Build history of the part. All positions in model axes, mm. A direction names the side the tool comes from. Give positions to 0.01 mm unless a question says otherwise; leave off trailing zeros. Order: outer loops, then holes, each group sorted by start corner. A loop starts at its lowest first (then second) coordinate and runs counter-clockwise, first axis right, second up. Notation, with made-up numbers: (-25.75, 23) -> (-10.75, 23) arc R22 ccw to (-10.75, 43) -> close; hole circle Ø9 at (28, -8). An arc over 180 degrees is marked (long way). One line per item, written item: value. Start each with the question number.
(1) Saw through at C-C on x = -5. Give the cut face in (y, z).
(2) Saw through at B-B on x = 5.5. Give the cut face in (y, z).
(3) Pin check, flat tips, straight feed: pin 1 (1.8 mm diameter, centred on x = 15.5, y = -1, fed in from +Z); pin 2 (10 mm diameter, centred on y = -3, z = 33, fed in from +X); pin 3 (3 mm diameter, centred on y = 1.5, z = 20.5, fed in from +X). Stop position of each tip, or through.
(4) Two-plate mould, pull along Y, no slides. Class faces 6 (the flat face through (6, 0, 19.55)), 7 (the flat face through (5, 0, 23)), 8 (the flat face through (0, 10, 6)): +Y half, -Y half, draft (parallel to the pull), parting line (faces both ways), or undercut.
(5) Saw through at D-D on z = 23.5. Give the cut face in (x, y), plus the area to 3 significant figures.
(6) Probe line 1 (X direction, y = 0, z = 1.7); line 2 (Y direction, x = -5, z = 3); line 3 (X direction, y = 4.5, z = 32). List the from-to ranges inside material, lowest first.
(7) Which spindle directions (+Z, -Z, +X, -X, +Y, -Y) get a long thin tool onto all of the face, cutting with end or side? Do faces 1 (the cylindrical face through (12.789, 1.933, 6.521)), 2 (the flat face through (-10, 0, 23)), 3 (the flat face through (15.437, 7.535, 23.21)), 4 (the flat face through (6, 0, 12.45)), 5 (the flat face through (18.4, 0.1, 8)). Say none if no direction does.
(8) Saw through at A-A on z = 30.5. Give the cut face in (x, y).
```python
from build123d import *

# Parameters (mm, degrees)
SKETCH1_W           = 40
SKETCH1_H           = 20
SKETCH1_R           = 1.65
BOSS_EXTRUDE1_DEPTH = 8
SKETCH3_W           = 3
SKETCH3_H           = 20
SKETCH3_W_2         = 6
BOSS_EXTRUDE2_DEPTH = 30
BOSS_EXTRUDE3_DEPTH = 20
SKETCH6_W           = 7
SKETCH6_H           = 10
SKETCH6_W_2         = 9
CUT_EXTRUDE2_DEPTH  = 30
SKETCH7_R           = 2.15
CUT_EXTRUDE3_DEPTH  = 6
CUT_EXTRUDE4_DEPTH  = 2.5
SKETCH10_R          = 3
CUT_EXTRUDE5_DEPTH  = 3


with BuildPart() as part:
    # Sketch1 → Boss-Extrude1 (new body)
    with BuildSketch(Plane.XY):
        Rectangle(SKETCH1_W, SKETCH1_H)
        with Locations((-5, 0)):
            Circle(SKETCH1_R, mode=Mode.SUBTRACT)
        with Locations((14.999778189, -0.094193404)):
            Circle(SKETCH1_R, mode=Mode.SUBTRACT)
    extrude(amount=BOSS_EXTRUDE1_DEPTH)

    # Sketch3 → Boss-Extrude2 (add)
    with BuildSketch(Plane.XY.offset(8)):
        with Locations((-11.5, 0)):
            Rectangle(SKETCH3_W, SKETCH3_H)
        with Locations((8, 0)):
            Rectangle(SKETCH3_W_2, SKETCH3_H)
    extrude(amount=BOSS_EXTRUDE2_DEPTH)

    # Sketch5 → Boss-Extrude3 (add)
    with BuildSketch(Plane(origin=(0, 10, 0), x_dir=(1, 0, 0), z_dir=(0, 1, 0))):
        Polygon((-20, -8), (-13, -38), (-13, -8), align=None)
        Polygon((20, -8), (11, -8), (11, -38), align=None)
    extrude(amount=-BOSS_EXTRUDE3_DEPTH)

    # Sketch6 → Cut-Extrude2 (cut)
    with BuildSketch(Plane.XY.offset(38)):
        with Locations((-16.5, 0)):
            Rectangle(SKETCH6_W, SKETCH6_H)
        with Locations((15.5, 0)):
            Rectangle(SKETCH6_W_2, SKETCH6_H)
    extrude(amount=-CUT_EXTRUDE2_DEPTH, mode=Mode.SUBTRACT)

    # Sketch7 → Cut-Extrude3 (cut)
    with BuildSketch(Plane(origin=(11, 0, 0), x_dir=(0, 0, -1), z_dir=(1, 0, 0))):
        with Locations(Location((-16, 0, 0), (0, 0, 90))):
            Circle(SKETCH7_R)
    extrude(amount=-CUT_EXTRUDE3_DEPTH, mode=Mode.SUBTRACT)

    # Sketch8 → Cut-Extrude4 (cut)
    with BuildSketch(Plane.ZY.offset(-5)):
        Polygon((19.55, 2.049593456), (16, 4.099186911), (12.45, 2.049593456), (12.45, -2.049593456), (16, -4.099186911), (19.55, -2.049593456), align=None)
    extrude(amount=-CUT_EXTRUDE4_DEPTH, mode=Mode.SUBTRACT)

    # Sketch10 → Cut-Extrude5 (cut)
    with BuildSketch(Plane.XY.offset(8)):
        with Locations((-5, 0)):
            Circle(SKETCH10_R)
        with Locations((14.999778189, -0.094193404)):
            Circle(SKETCH10_R)
    extrude(amount=-CUT_EXTRUDE5_DEPTH, mode=Mode.SUBTRACT)


solid = part.part
```
Results below:
1. outline: (-10, 0) -> (-1.65, 0) -> (-1.65, 5) -> (-3, 5) -> (-3, 8) -> (-10, 8) -> close; (1.65, 0) -> (10, 0) -> (10, 8) -> (3, 8) -> (3, 5) -> (1.65, 5) -> close
2. outline: (-10, 0) -> (10, 0) -> (10, 38) -> (-10, 38) -> close; hole (-4.1, 16) -> (-2.05, 12.45) -> (2.05, 12.45) -> (4.1, 16) -> (2.05, 19.55) -> (-2.05, 19.55) -> close
3. pin 1: stops at z = 5
3. pin 2: stops at x = 13.87
3. pin 3: stops at x = 11
4. face 6: undercut
4. face 7: draft
4. face 8: +Y half
5. outline: (-16.38, -10) -> (-10, -10) -> (-10, 10) -> (-16.38, 10) -> (-16.38, 5) -> (-13, 5) -> (-13, -5) -> (-16.38, -5) -> close; (5, -10) -> (15.35, -10) -> (15.35, -5) -> (11, -5) -> (11, 5) -> (15.35, 5) -> (15.35, 10) -> (5, 10) -> close
5. area: 257 mm²
6. line 1: x = -20 to -6.65, -3.35 to 13.35, 16.65 to 20
6. line 2: y = -10 to -1.65, 1.65 to 10
6. line 3: x = -13 to -10, 5 to 11
7. face 1: +Z
7. face 2: +Z, +Y, -Y
7. face 3: +Z, +X, +Y, -Y
7. face 4: none
7. face 5: +Z, +X
8. outline: (-14.75, -10) -> (-10, -10) -> (-10, 10) -> (-14.75, 10) -> (-14.75, 5) -> (-13, 5) -> (-13, -5) -> (-14.75, -5) -> close; (5, -10) -> (13.25, -10) -> (13.25, -5) -> (11, -5) -> (11, 5) -> (13.25, 5) -> (13.25, 10) -> (5, 10) -> close
